from build123d import *

# Parameters (mm, degrees)
SKETCH1_W           = 80
SKETCH1_H           = 23
BOSS_EXTRUDE3_DEPTH = 10
SKETCH4_W           = 50
SKETCH4_H           = 14.8
CUT_EXTRUDE1_DEPTH  = 10
SKETCH6_R           = 1.5
CUT_EXTRUDE5_DEPTH  = 10
SKETCH7_W           = 33
SKETCH7_H           = 8.2
BOSS_EXTRUDE4_DEPTH = 5
SKETCH5_R           = 1.5
CUT_EXTRUDE2_DEPTH  = 19


with BuildPart() as part:
    # Sketch1 → Boss-Extrude3 (new body)
    with BuildSketch(Plane.XY):
        with Locations((40, 11.5)):
            Rectangle(SKETCH1_W, SKETCH1_H)
    extrude(amount=BOSS_EXTRUDE3_DEPTH)

    # Sketch4 → Cut-Extrude1 (cut)
    with BuildSketch(Plane.XY.offset(10)):
        with Locations((40, 15.6)):
            Rectangle(SKETCH4_W, SKETCH4_H)
    extrude(amount=-CUT_EXTRUDE1_DEPTH, mode=Mode.SUBTRACT)

    # Sketch6 → Cut-Extrude5 (cut)
    with BuildSketch(Plane.XY.offset(10)):
        with Locations((5, 18)):
            Circle(SKETCH6_R)
        with Locations((5, 11)):
            Circle(SKETCH6_R)
        with Locations((75, 11)):
            Circle(SKETCH6_R)
        with Locations((75, 18)):
            Circle(SKETCH6_R)
    extrude(amount=-CUT_EXTRUDE5_DEPTH, mode=Mode.SUBTRACT)

    # Sketch7 → Boss-Extrude4 (add)
    with BuildSketch(Plane(origin=(0, 0, 0), x_dir=(-1, 0, 0), z_dir=(0, 0, -1))):
        with Locations((-40, 4.1)):
            Rectangle(SKETCH7_W, SKETCH7_H)
    extrude(amount=BOSS_EXTRUDE4_DEPTH)

    # Sketch5 → Cut-Extrude2 (cut)
    with BuildSketch(Plane.XY.offset(10)):
        with Locations((32.25, 4.2)):
            Circle(SKETCH5_R)
        with Locations((47.75, 4.2)):
            Circle(SKETCH5_R)
    extrude(amount=-CUT_EXTRUDE2_DEPTH, mode=Mode.SUBTRACT)


solid = part.part
The listing builds one solid part. Answer for the finished solid, in the listing's coordinates (mm). A direction names the side the tool comes from. Give positions to 0.01 mm unless a question says otherwise; leave off trailing zeros. Write each loop counter-clockwise with the first axis right and the second up, starting at its lowest first coordinate (ties: lowest second). Pieces come first, ordered by that corner, then holes.
Item 1: Section A-A, the plane x = 5 is taken. Write down the section's boundary in (y, z), plus the area to 3 significant figures.
Item 2: Determine the mould class of faces 5 (the flat face through (40, 4, -5)), 6 (the flat face through (39, 7, 10)), 7 (the flat face through (40, 8.2, 3)) for opening direction Z: released by +Z, released by -Z, zero draft, split by the parting line, or undercut.
Item 3: Section B-B, the plane y = 4.2 is taken. Write down the section's boundary in (x, z), plus the area to 3 significant figures.
Item 4: Section D-D, the plane z = 2 is taken. Write down the section's boundary in (x, y), plus the area to 3 significant figures.
Item 5: Which of the six approach directions +Z, -Z, +X, -X, +Y, -Y give full straight-line access (tool end or side, diameter ignored) to faces 1 (the flat face through (23.5, 4, -2)), 2 (the flat face through (71, 12, 0)), 3 (the cylindrical face through (46.25, 4.27, 2.61)), 4 (the flat face through (65, 15, 5))?
Item 6: Flat-ended cylindrical pins translate along their axes: P1, Ø11.5, axis at x = 73.5, y = 14.5, coming from the -Z side; P2, Ø2.5, axis at y = 5.5, z = -2.5, coming from the +X side; P3, Ø1.8, axis at x = 75, y = 11, coming from the -Z side; P4, Ø5, axis at y = 7.5, z = -3, coming from the -X side. Find the tip coordinate at first contact, or state that the pin passes through.
Item 7: Section C-C, the plane y = 21.75 is taken. Write down the section's boundary in (x, z).
Item 8: Find the intervals of material crossed by line 1 along Y through (x, z) = (5, 4); line 2 along X through (y, z) = (16, 1.25); line 3 along X through (y, z) = (10, 9.25), in increasing order.
Completed:
1. outline: (0, 0) - (9.5, 0) - (9.5, 10) - (0, 10) - close; (12.5, 0) - (16.5, 0) - (16.5, 10) - (12.5, 10) - close; (19.5, 0) - (23, 0) - (23, 10) - (19.5, 10) - close
1. area: 170 mm2
2. face 5: released by -Z
2. face 6: released by +Z
2. face 7: zero draft
3. outline: (0, 0) - (23.5, 0) - (23.5, -5) - (30.75, -5) - (30.75, 10) - (0, 10) - close; (33.75, -5) - (46.25, -5) - (46.25, 10) - (33.75, 10) - close; (49.25, -5) - (56.5, -5) - (56.5, 0) - (80, 0) - (80, 10) - (49.25, 10) - close
3. area: 875 mm2
4. outline: (0, 0) - (80, 0) - (80, 23) - (65, 23) - (65, 8.2) - (15, 8.2) - (15, 23) - (0, 23) - close; hole circle Ø3 at (5, 11); hole circle Ø3 at (5, 18); hole circle Ø3 at (32.25, 4.2); hole circle Ø3 at (47.75, 4.2); hole circle Ø3 at (75, 11); hole circle Ø3 at (75, 18)
4. area: 1,060 mm2
5. face 1: -Z, -X, +Y, -Y
5. face 2: -Z, +X, +Y, -Y
5. face 3: +Z, -Z
5. face 4: +Z, -Z, +Y
6. P1: stops at z = 0
6. P2: stops at x = 56.5
6. P3: passes through
6. P4: stops at x = 23.5
7. outline: (0, 0) - (15, 0) - (15, 10) - (0, 10) - close; (65, 0) - (80, 0) - (80, 10) - (65, 10) - close
8. line 1: y = 0 to 9.5, 12.5 to 16.5, 19.5 to 23
8. line 2: x = 0 to 15, 65 to 80
8. line 3: x = 0 to 3.88, 6.12 to 15, 65 to 73.88, 76.12 to 80
